Could you check a few things on this model? Use its own coordinates, in mm. Face numbers are marked on the shaded views. A direction names the side the tool comes from. Round coordinates to 2 decimals unless told otherwise and drop trailing zeros. Order: outer loops, then holes, each group sorted by start corner. A loop starts at its lowest first (then second) coordinate and runs counter-clockwise, first axis right, second up. Notation, with made-up numbers: M -2.5,89 L 13.5,89 A20 cw 13.5,110 Z; hole C 70.25,45.25 d11. An arc over 180 degrees is marked long. Write each question's results on one line, items separated by ' | '. Start each with the question number.
1. For the marked faces 4 and 5, which set-ups out of +Z, -Z, +X, -X, +Y, -Y let a thin tool reach every point of the face, with its end or its side?
2. Suppose I cut it at A-A on x = 1. Write out the boundary of the cut face in (y, z) (3 decimals), and give its area (3 significant figures).
3. Suppose I cut it at B-B on z = 8.75. Write out the boundary of the cut face in (x, y) (3 decimals).
4. Suppose I cut it at C-C on y = 10. Write out the boundary of the cut face in (x, z) (3 decimals), and give its area (3 significant figures).
5. I'm going to push a flat-ended pin straight in: pin 1 (2 mm diameter, centred on x = 9.5, y = 18, fed in from -Z) (3 decimals). Where does the tip first touch, or does it pass through?
6. Suppose I cut it at D-D on z = -1. Write out the boundary of the cut face in (x, y) (3 decimals).
7. Please list where these lines run through material, in increasing order: L1, parallel to X at y = 11, z = -6 (3 decimals); L2, parallel to Z at x = -10, y = 12 (3 decimals); L3, parallel to Y at x = 0, z = 12.25.
8. We'd pull the mould along X, two halves only. Please class the marked faces 1, 2 and 3: released by +X, released by -X, zero draft, split by the parting line, or undercut.
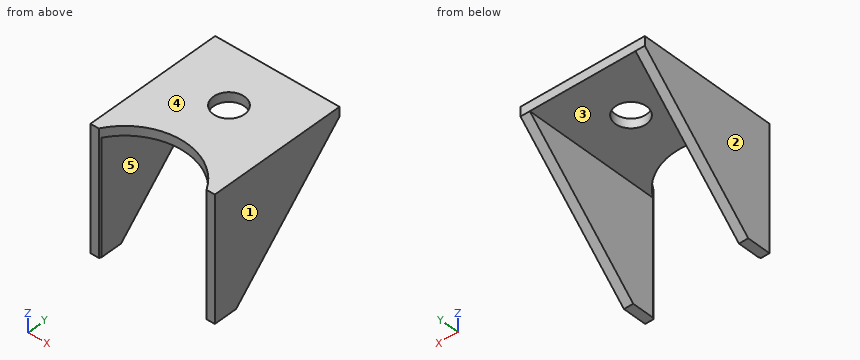
from build123d import *

# Parameters (mm, degrees)
BOSS_EXTRUDE1_DEPTH = 34.671
CUT_EXTRUDE1_DEPTH  = 45.816606755
SKETCH3_R           = 3.175
CUT_EXTRUDE2_DEPTH  = 45.816606755
CUT_EXTRUDE3_DEPTH  = 45.816606755


with BuildPart() as part:
    # Sketch1 → Boss-Extrude1 (new body)
    with BuildSketch(Plane(origin=(0, 0, 0), x_dir=(1, 0, 0), z_dir=(0, 1, 0))):
        Polygon((-12.7, 12.7), (-12.7, -12.7), (12.7, -12.7), (12.7, 12.7), (10.795, 12.7), (10.795, -10.795), (-10.795, -10.795), (-10.795, 12.7), align=None)
    extrude(amount=BOSS_EXTRUDE1_DEPTH)

    # Sketch2 → Cut-Extrude1 (cut, through all)
    with BuildSketch(Plane.ZY.offset(12.7)):
        Polygon((-12.7, 11.176), (10.795, 34.671), (-12.7, 34.671), align=None)
    extrude(amount=-CUT_EXTRUDE1_DEPTH, mode=Mode.SUBTRACT)

    # Sketch3 → Cut-Extrude2 (cut, through all)
    with BuildSketch(Plane.XY.offset(12.7)):
        with Locations((0, 23.6855)):
            Circle(SKETCH3_R)
    extrude(amount=-CUT_EXTRUDE2_DEPTH, mode=Mode.SUBTRACT)

    # Sketch4 → Cut-Extrude3 (cut, through all)
    with BuildSketch(Plane.XY.offset(12.7)):
        with BuildLine():
            Line((-12.7, 0), (12.7, 0))
            Line((12.7, 0), (12.7, 6.35))
            Line((12.7, 6.35), (10.998522628, 6.35))
            ThreePointArc((10.998522628, 6.35), (0, 12.7), (-10.998522628, 6.35))
            Line((-10.998522628, 6.35), (-12.7, 6.35))
            Line((-12.7, 6.35), (-12.7, 0))
        make_face()
    extrude(amount=-CUT_EXTRUDE3_DEPTH, mode=Mode.SUBTRACT)


solid = part.part
Filled sheet:
1) face 4: +Z, +X, -X, +Y, -Y | face 5: -Z, +Y, -Y
2) outline: M 12.661,10.795 L 20.672,10.795 L 20.672,12.7 L 12.661,12.7 Z; M 26.699,10.795 L 34.671,10.795 L 34.671,12.7 L 26.699,12.7 Z | area: 30.4 mm^2
3) outline: M -12.7,6.35 L -10.999,6.35 A12.7 cw -10.795,6.69 L -10.795,32.626 L -12.7,32.626 Z; M 10.795,6.69 A12.7 cw 10.999,6.35 L 12.7,6.35 L 12.7,32.626 L 10.795,32.626 Z
4) outline: M -12.7,-12.7 L -10.795,-12.7 L -10.795,10.795 L -7.829,10.795 L -7.829,12.7 L -12.7,12.7 Z; M 7.829,10.795 L 10.795,10.795 L 10.795,-12.7 L 12.7,-12.7 L 12.7,12.7 L 7.829,12.7 Z | area: 108 mm^2
5) pin 1: stops at z = 10.795
6) outline: M -12.7,6.35 L -10.999,6.35 A12.7 cw -10.795,6.69 L -10.795,22.876 L -12.7,22.876 Z; M 10.795,6.69 A12.7 cw 10.999,6.35 L 12.7,6.35 L 12.7,22.876 L 10.795,22.876 Z
7) L1: x = -12.7 to -10.795, 10.795 to 12.7 | L2: z = 10.795 to 12.7 | L3: y = 12.7 to 20.51, 26.86 to 34.67
8) face 1: released by +X | face 2: released by -X | face 3: undercut
